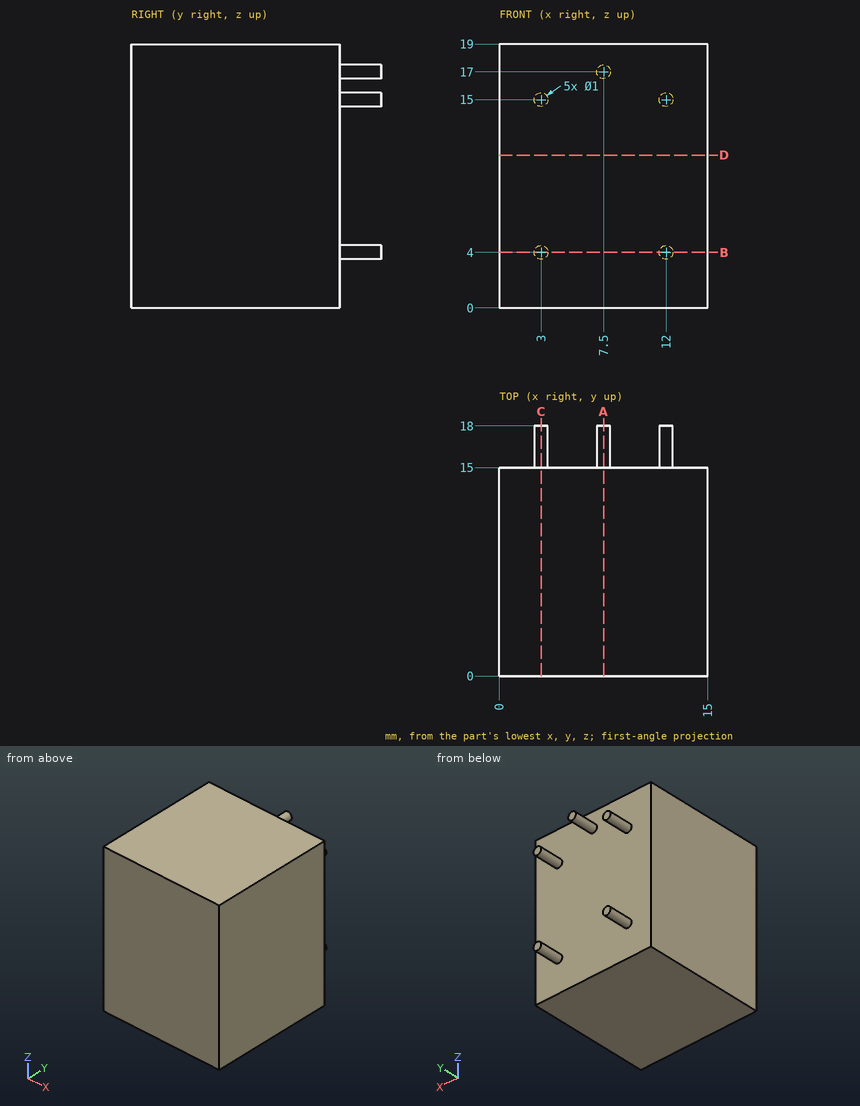
The figure shows three views and two pictorial views of one solid part (mm, origin at its lowest corner). Answer the questions. Coordinates: 2 decimals unless noted, no trailing zeros. Loops run counter-clockwise (first coordinate to the right, second up) from the corner with the lowest first, then second, coordinate; pieces in that order, holes last. Notation, with made-up numbers: M 57,-4.75 L 90,-4.75 A16 ccw 90,19.25 Z; hole C -15,-17 d10. An arc over 180 degrees is marked long. Answer as CSV lines item,"result". Start each with the question number.
(1) Find the intervals of material crossed by L1, parallel to Y at x = 2, z = 14.25; L2, parallel to Z at x = 11.75, y = 16.75, in increasing order. Write a range as [from, to].
(2) The part is cut by section B-B (z = 4). Give the vertices of the cut face in (x, y).
(3) The part is cut by section A-A (x = 7.5). Give the vertices of the cut face in (y, z).
(4) Given pin 1 (7.5 mm diameter, centred on x = 7, z = 8.5, fed in from +Y); pin 2 (1 mm diameter, centred on y = 16, z = 12, fed in from +X), each flat-ended and moving along its own axis, determine where each tip first touches the part or whether it passes through.
(5) The part is cut by section D-D (z = 11). Give the vertices of the cut face in (x, y), and give its area (3 significant figures).
(6) The part is cut by section C-C (x = 3). Give the vertices of the cut face in (y, z).
Determined:
1,L1,"[0, 15]"
1,L2,"[3.57, 4.43], [14.57, 15.43]"
2,outline,"M 0,0 L 15,0 L 15,15 L 12.5,15 L 12.5,18 L 11.5,18 L 11.5,15 L 3.5,15 L 3.5,18 L 2.5,18 L 2.5,15 L 0,15 Z"
3,outline,"M 0,0 L 15,0 L 15,16.5 L 18,16.5 L 18,17.5 L 15,17.5 L 15,19 L 0,19 Z"
4,pin 1,"y = 15"
4,pin 2,"through"
5,outline,"M 0,0 L 15,0 L 15,15 L 0,15 Z"
5,area,"225 mm2"
6,outline,"M 0,0 L 15,0 L 15,3.5 L 18,3.5 L 18,4.5 L 15,4.5 L 15,14.5 L 18,14.5 L 18,15.5 L 15,15.5 L 15,19 L 0,19 Z"
